```python
from build123d import *

# Parameters (mm, degrees)
BOSS_EXTRUDE1_DEPTH = 3
BOSS_EXTRUDE2_DEPTH = 3
FILLET1_R           = 3
SKETCH4_R           = 1.25
CUT_EXTRUDE1_DEPTH  = 4


with BuildPart() as part:
    # Sketch1 → Boss-Extrude1 (new body)
    with BuildSketch(Plane(origin=(0, 0, 0), x_dir=(1, 0, 0), z_dir=(0, 1, 0))):
        with BuildLine():
            Line((29.1, -16), (29.1, -12))
            Line((29.1, -12), (28, -12))
            Line((28, -12), (28, -2))
            Line((28, -2), (25.57587166, 6.937203242))
            ThreePointArc((25.57587166, 6.937203242), (16.099908604, 21.048585296), (0, 26.5))
            Line((0, 26.5), (0, 32.5))
            ThreePointArc((0, 32.5), (19.745170929, 25.814302721), (31.366635055, 8.507890769))
            Line((31.366635055, 8.507890769), (34, -1.200719678))
            Line((34, -1.200719678), (34, -12))
            Line((34, -12), (32.9, -12))
            Line((32.9, -12), (32.9, -21))
            Line((32.9, -21), (33.4, -22))
            Line((33.4, -22), (33.9, -22.5))
            Line((33.9, -22.5), (33.9, -23.5))
            Line((33.9, -23.5), (32.4, -25))
            Line((32.4, -25), (30.9, -25))
            Line((30.9, -25), (29.1, -16))
        make_face()
    extrude(amount=BOSS_EXTRUDE1_DEPTH)

    # Sketch3 → Boss-Extrude2 (add)
    with BuildSketch(Plane(origin=(0, 0, 0), x_dir=(1, 0, 0), z_dir=(0, 1, 0))):
        with BuildLine():
            Line((28, -6), (28, -12))
            ThreePointArc((28, -12), (25, -9), (28, -6))
        make_face()
    extrude(amount=BOSS_EXTRUDE2_DEPTH)

    # Fillet1
    fillet1_edges = [part.edges().sort_by_distance(p)[0] for p in [
        (28, 1.5, 6),
    ]]
    fillet(fillet1_edges, radius=FILLET1_R)

    # Sketch4 → Cut-Extrude1 (cut, through all)
    with BuildSketch(Plane(origin=(0, 3, 0), x_dir=(1, 0, 0), z_dir=(0, 1, 0))):
        with Locations((28, -9)):
            Circle(SKETCH4_R)
    extrude(amount=-CUT_EXTRUDE1_DEPTH, mode=Mode.SUBTRACT)

    # Mirror1: part across plane


with BuildPart() as part_1:
    add(part.part)
    add(part.part.mirror(Plane(origin=(0, 0, 0), x_dir=(0, 0, 1), z_dir=(1, 0, 0))))


solid = part_1.part
```
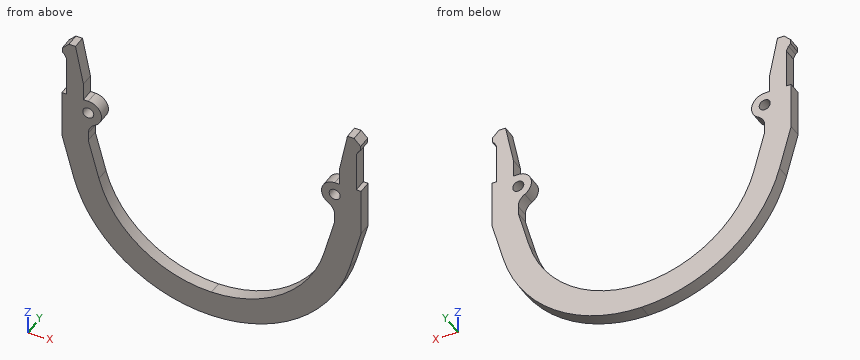
Source: CAD feature listing. Evaluate the final solid. Frame: model axes, mm. Round coordinates to 2 decimals unless told otherwise and drop trailing zeros. Loops run counter-clockwise (first coordinate to the right, second up) from the corner with the lowest first, then second, coordinate; pieces in that order, holes last. Notation, with made-up numbers: M 56.25,-40 L 110.25,-40 A22 ccw 110.25,-9 Z; hole C 82,-34.5 d6. An arc over 180 degrees is marked long. Use a Markdown table: item, result. Add a question column.
1. Section query B-B on z = 0. Return the cut outline in (x, y).
2. Section query A-A on z = 9. Return the cut outline in (x, y).
3. Section query D-D on x = -5.5. Return the cut outline in (y, z), then the cut area to 3 significant figures.
4. Contact query for flat-ended pins moving along their axis: P1, Ø1.5, axis at y = 1, z = 14, coming from the +X side; P2, Ø1.2, axis at x = 33.5, y = 1, coming from the +Z side; P3, Ø5, axis at x = 20.5, z = 8.5, coming from the -Y side; P4, Ø0.6, axis at x = -33.5, y = 1.5, coming from the +Z side. Output: stop coordinate, or through.
5. Line query: line 1 (X direction, y = 2.2, z = 9); line 2 (X direction, y = 1, z = 2); line 3 (Z direction, x = 29, y = 0.8). Output: solid intervals per line, ascending.
6. Section query C-C on y = 0.7. Give the number of separate pieces and of enclosed holes in the cut face, then the cut area to 3 significant figures.
Reported:
| question | item | result |
|---|---|---|
| 1 | outline | M -33.67,0 L -27.46,0 L -27.46,3 L -33.67,3 Z; M 27.46,0 L 33.67,0 L 33.67,3 L 27.46,3 Z |
| 2 | outline | M -34,0 L -29.25,0 L -29.25,3 L -34,3 Z; M -26.75,0 L -25,0 L -25,3 L -26.75,3 Z; M 25,0 L 26.75,0 L 26.75,3 L 25,3 Z; M 29.25,0 L 34,0 L 34,3 L 29.25,3 Z |
| 3 | outline | M 0,-32.03 L 3,-32.03 L 3,-25.92 L 0,-25.92 Z |
| 3 | area | 18.3 mm² |
| 4 | P1 | stops at x = 32.9 |
| 4 | P2 | stops at z = 24.5 |
| 4 | P3 | passes through |
| 4 | P4 | stops at z = 24.2 |
| 5 | line 1 | x = -34 to -29.25, -26.75 to -25, 25 to 26.75, 29.25 to 34 |
| 5 | line 2 | x = -34 to -28, 28 to 34 |
| 5 | line 3 | z = -14.67 to 8.25, 9.75 to 12 |
| 6 | separate pieces | 1 |
| 6 | enclosed holes | 2 |
| 6 | area | 810 mm² |
